Geometry check sheet. Reference: the model listing, model coordinates, mm. Coordinates: 2 decimals unless noted, no trailing zeros. Order: outer loops, then holes, each group sorted by start corner. A loop starts at its lowest first (then second) coordinate and runs counter-clockwise, first axis right, second up.
```python
from build123d import *

# Parameters (mm, degrees)
BOSS_EXTRUDE1_DEPTH       = 6.35
F_4_CLEARANCE_HOLE1_D     = 3.2639
F_4_CLEARANCE_HOLE1_DEPTH = 12.7
F_4_CLEARANCE_HOLE1_TIP   = 0.980574487
FILLET1_R                 = 3.175


with BuildPart() as part:
    # Sketch1 → Boss-Extrude1 (new body)
    with BuildSketch(Plane.XY):
        Polygon((-38.1, -57.15), (41.275, -19.05), (41.275, 6.35), (-38.1, 6.35), align=None)
    extrude(amount=BOSS_EXTRUDE1_DEPTH)

    # #4 Clearance Hole1
    with Locations(Plane.XY.offset(6.35)):
        with Locations((-34.29, 0), (-18.415, 0), (34.925, 0), (-34.29, -44.45)):
            Hole(F_4_CLEARANCE_HOLE1_D / 2, depth=F_4_CLEARANCE_HOLE1_DEPTH)
            with Locations((0, 0, -(F_4_CLEARANCE_HOLE1_DEPTH + F_4_CLEARANCE_HOLE1_TIP / 2))):  # 118° drill point
                Cone(0, F_4_CLEARANCE_HOLE1_D / 2, F_4_CLEARANCE_HOLE1_TIP, mode=Mode.SUBTRACT)

    # Fillet1
    fillet1_edges = [part.edges().sort_by_distance(p)[0] for p in [
        (41.275, -19.05, 3.175),
        (-38.1, -57.15, 3.175),
        (-38.1, 6.35, 3.175),
        (41.275, 6.35, 3.175),
    ]]
    fillet(fillet1_edges, radius=FILLET1_R)


solid = part.part
```
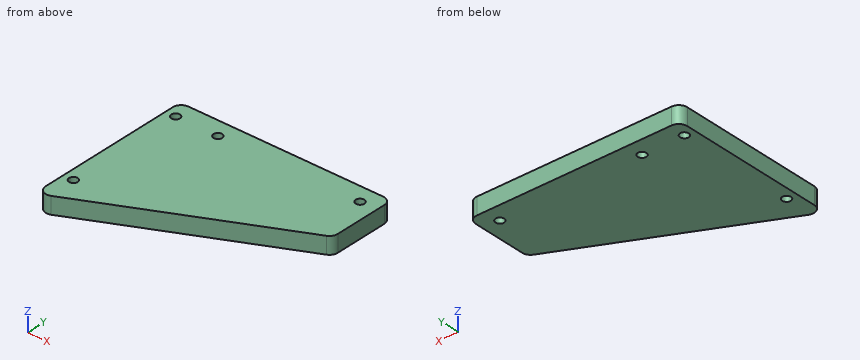
Item 1: Sectioned sample at D-D (x = 35). Record the cut outline in (y, z), and give its area (3 significant figures).
Item 2: Thickness scan on line 1 along Y through (x, z) = (-34.29, 4.75); line 2 along Y through (x, z) = (-17.5, 3.75); line 3 along X through (y, z) = (-50, 6). Record the ranges inside material, lowest first.
Item 3: Sectioned sample at A-A (y = 0). Record the cut outline in (x, z) (3 decimals).
Item 4: Sectioned sample at B-B (z = 4.25). Record the cut outline in (x, y) (3 decimals).
Item 5: Depth check by flat-ended pin: P1, Ø2, axis at x = -4, y = -25.5, coming from the -Z side; P2, Ø3, axis at x = -23, z = 1, coming from the -Y side. Enter the tip coordinate at first touch or a pass-through.
Item 6: Sectioned sample at C-C (y = -44.45). Record the cut outline in (x, z).
Geometry check:
1. outline: (-22.06, 0) - (-1.63, 0) - (-1.63, 6.35) - (-22.06, 6.35) - close; (1.63, 0) - (6.35, 0) - (6.35, 6.35) - (1.63, 6.35) - close
1. area: 160 mm2
2. line 1: y = -55.22 to -46.08, -42.82 to -1.63, 1.63 to 6.35
2. line 2: y = -47.26 to -1.35, 1.35 to 6.35
2. line 3: x = -38.1 to -23.2
3. outline: (-38.1, 0) - (-35.922, 0) - (-35.922, 6.35) - (-38.1, 6.35) - close; (-32.658, 0) - (-20.047, 0) - (-20.047, 6.35) - (-32.658, 6.35) - close; (-16.783, 0) - (33.293, 0) - (33.293, 6.35) - (-16.783, 6.35) - close; (36.557, 0) - (41.275, 0) - (41.275, 6.35) - (36.557, 6.35) - close
4. outline: (-38.1, -52.104) arc R3.175 ccw to (-33.551, -54.967) - (39.474, -19.915) arc R3.175 ccw to (41.275, -17.052) - (41.275, 3.175) arc R3.175 ccw to (38.1, 6.35) - (-34.925, 6.35) arc R3.175 ccw to (-38.1, 3.175) - close; hole circle Ø3.264 at (-34.29, -44.45); hole circle Ø3.264 at (-34.29, 0); hole circle Ø3.264 at (-18.415, 0); hole circle Ø3.264 at (34.925, 0)
5. P1: stops at z = 0
5. P2: stops at y = -50.62
6. outline: (-38.1, 0) - (-35.92, 0) - (-35.92, 6.35) - (-38.1, 6.35) - close; (-32.66, 0) - (-11.64, 0) - (-11.64, 6.35) - (-32.66, 6.35) - close
